Read the model definition and answer for the solid it produces. Units are mm, in the model's axes. A direction names the side the tool comes from. Give positions to 0.01 mm unless a question says otherwise; leave off trailing zeros. Order: outer loops, then holes, each group sorted by start corner. A loop starts at its lowest first (then second) coordinate and runs counter-clockwise, first axis right, second up.
Item 1: A cutting plane is placed at A-A (x = 0). Write down the section's boundary in (y, z), plus the area to 3 significant figures.
Item 2: Find the intervals of material crossed by line 1 along Y through (x, z) = (12.5, 76.5), in increasing order.
Item 3: A cutting plane is placed at B-B (x = 16). Write down the section's boundary in (y, z), plus the area to 3 significant figures.
Item 4: The mould has two halves that part along Z. Classify faces 1 (the face through (-0.833, 29.986, 38.252)), 2 (the face through (0, 31, 34)), 3 (the face through (0, 0, 0)): +Z half, -Z half, draft (parallel to the pull), parting line (faces both ways), or undercut.
Item 5: Which of the six approach directions +Z, -Z, +X, -X, +Y, -Y give full straight-line access (tool end or side, diameter ignored) to faces 4 (the face through (18.5, 0, 40)), 5 (the face through (-0.833, 29.986, 58.252))?
from build123d import *

# Parameters (mm, degrees)
SKETCH_1_W      = 37
SKETCH_1_H      = 58
EXTRUDE_1_DEPTH = 81
SKETCH_3_R      = 3.842727579
EXTRUDE_2_DEPTH = 2


with BuildPart() as part:
    # 草图1 → 凸台-拉伸1 (new body)
    with BuildSketch(Plane.XY):
        Rectangle(SKETCH_1_W, SKETCH_1_H)
    extrude(amount=EXTRUDE_1_DEPTH)

    # 草图3 → 凸台-拉伸2 (add)
    with BuildSketch(Plane(origin=(0, 29, 0), x_dir=(1, 0, 0), z_dir=(0, 1, 0))):
        with Locations((0, -14.500282865)):
            Circle(SKETCH_3_R)
        with Locations((0, -34.500282865)):
            Circle(SKETCH_3_R)
        with Locations((0, -54.500282865)):
            Circle(SKETCH_3_R)
    extrude(amount=EXTRUDE_2_DEPTH)


solid = part.part
Response values:
1. outline: (-29, 0) - (29, 0) - (29, 10.66) - (31, 10.66) - (31, 18.34) - (29, 18.34) - (29, 30.66) - (31, 30.66) - (31, 38.34) - (29, 38.34) - (29, 50.66) - (31, 50.66) - (31, 58.34) - (29, 58.34) - (29, 81) - (-29, 81) - close
1. area: 4,740 mm2
2. line 1: y = -29 to 29
3. outline: (-29, 0) - (29, 0) - (29, 81) - (-29, 81) - close
3. area: 4,700 mm2
4. face 1: undercut
4. face 2: draft
4. face 3: -Z half
5. face 4: +Z, -Z, +X, +Y, -Y
5. face 5: +Y
